Input: part model. Units: mm. Frame: model coordinates. Coordinates: 2 decimals unless noted, no trailing zeros. Loops run counter-clockwise (first coordinate to the right, second up) from the corner with the lowest first, then second, coordinate; pieces in that order, holes last. Notation, with made-up numbers: (45.5, 84) - (103.5, 84) arc R20 ccw to (103.5, 99) - close; hole circle Ø5 at (-20.75, -11). An arc over 180 degrees is marked (long way). Use one line per item in the form item = value.
from build123d import *

# Parameters (mm, degrees)
SKETCH1_W                   = 259.842
SKETCH1_H                   = 155.702
SKETCH1_W_2                 = 183.642
SKETCH1_H_2                 = 79.502
BOSS_EXTRUDE1_DEPTH         = 6.35
F_1_4_0_25_DIAMETER_SLOT1_D = 6.35


with BuildPart() as part:
    # Sketch1 → Boss-Extrude1 (new body)
    with BuildSketch(Plane.XY):
        with Locations((91.821, 39.751)):
            Rectangle(SKETCH1_W, SKETCH1_H)
        with Locations((91.821, 39.751)):
            Rectangle(SKETCH1_W_2, SKETCH1_H_2, mode=Mode.SUBTRACT)
    extrude(amount=BOSS_EXTRUDE1_DEPTH)

    # 1/4 (0.25) Diameter Slot1 (through all)
    with Locations(Plane.XY.offset(6.35)):
        with Locations((29.067540373, 98.907455137), (93.740319595, 98.907455137), (162.414380138, 98.907455137), (162.414380138, -18.916352314), (93.740319595, -18.916352314), (29.067540373, -18.916352314)):
            Hole(F_1_4_0_25_DIAMETER_SLOT1_D / 2)


solid = part.part
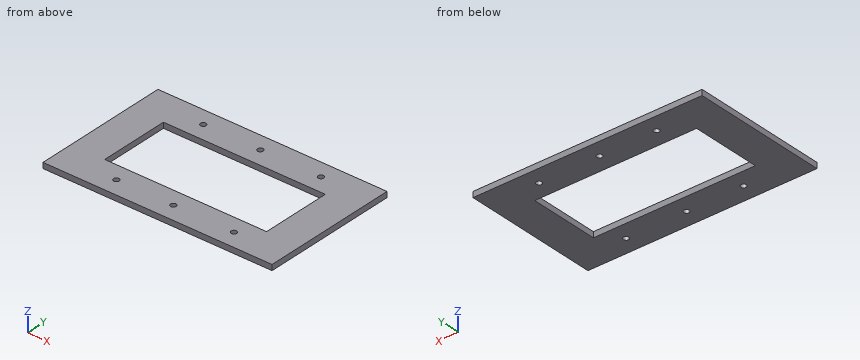
Q1. First-contact query: P1, Ø5, axis at x = 162.41, y = 98.91, coming from the -Z side. Flat tip, straight axial feed; report the tip coordinate or a pass-through.
Check values:
P1 = through
Q2. Cut plane C-C, the plane z = 1. Return loops of the section in (x, y) (3 decimals), then the cut area to 3 significant figures.
Check values:
outline = (-38.1, -38.1) - (221.742, -38.1) - (221.742, 117.602) - (-38.1, 117.602) - close; hole (0, 0) - (183.642, 0) - (183.642, 79.502) - (0, 79.502) - close; hole circle Ø6.35 at (29.068, -18.916); hole circle Ø6.35 at (29.068, 98.907); hole circle Ø6.35 at (93.74, -18.916); hole circle Ø6.35 at (93.74, 98.907); hole circle Ø6.35 at (162.414, -18.916); hole circle Ø6.35 at (162.414, 98.907)
area = 25,700 mm²
Q3. Ray query, line 1 along Y through (x, z) = (136, 5.75); line 2 along X through (y, z) = (-21, 3.75); line 3 along X through (y, z) = (44, 5). Return the intervals inside material, ascending. Write a range as [from, to].
Check values:
line_1 = [-38.1, 0], [79.5, 117.6]
line_2 = [-38.1, 26.67], [31.46, 91.34], [96.14, 160.02], [164.81, 221.74]
line_3 = [-38.1, 0], [183.64, 221.74]
Q4. Cut plane B-B, the plane y = 29. Return loops of the section in (x, z).
Check values:
outline = (-38.1, 0) - (0, 0) - (0, 6.35) - (-38.1, 6.35) - close; (183.64, 0) - (221.74, 0) - (221.74, 6.35) - (183.64, 6.35) - close
Q5. Cut plane A-A, the plane x = 14.5. Return loops of the section in (y, z).
Check values:
outline = (-38.1, 0) - (0, 0) - (0, 6.35) - (-38.1, 6.35) - close; (79.5, 0) - (117.6, 0) - (117.6, 6.35) - (79.5, 6.35) - close
